Autodesk Inventor part; units mm, degrees
ref_plane "YZ Plane" through (0, 0, 0) normal (1, 0, 0) x (0, 1, 0)
ref_plane "XZ Plane" through (0, 0, 0) normal (0, 1, 0) x (-1, 0, 0)
ref_plane "XY Plane" through (0, 0, 0) normal (0, 0, 1) x (1, 0, 0)
sketch "Skizze1" plane through (0, 0, 0) normal (1, 0, 0) x (0, 1, 0)
  line L0 (12.7735, 187.5054) -> (12.7735, 177.5054) construction
  line L1 (12.7735, 177.5054) -> (95.7735, 177.5054) construction
  line L2 (95.7735, 177.5054) -> (95.7735, 203.5054) construction
  line L3 (91.4537, 203.5054) -> (93.2735, 198.5054) construction
  line L4 (95.7735, 203.5054) -> (80.7735, 203.5054) construction
  line L5 (93.2735, 198.5054) -> (83.2735, 198.5054) construction
  line L6 (83.2735, 198.5054) -> (85.0934, 203.5054) construction
  line L7 (80.7735, 203.5054) -> (80.7735, 187.5054) construction
  line L8 (80.7735, 187.5054) -> (12.7735, 187.5054) construction
  line L9 (12.7735, 187.5054) -> (12.7735, 177.5054) construction
  line L10 (15.2735, 182.5054) -> (17.0934, 187.5054) construction
  line L11 (25.2735, 182.5054) -> (15.2735, 182.5054) construction
  line L12 (23.4537, 187.5054) -> (25.2735, 182.5054) construction
  line L13 (95.7735, 177.5054) -> (95.7735, 203.4054)
  line L14 (95.7735, 203.4054) -> (91.5965, 203.4054)
  line L15 (91.5965, 203.4054) -> (93.4163, 198.4054)
  line L16 (93.4163, 198.4054) -> (83.1307, 198.4054)
  line L17 (83.1307, 198.4054) -> (84.9506, 203.4054)
  line L18 (84.9506, 203.4054) -> (80.8735, 203.4054)
  line L19 (80.8735, 203.4054) -> (80.8735, 187.4054)
  line L20 (80.8735, 187.4054) -> (23.5965, 187.4054)
  line L21 (23.5965, 187.4054) -> (25.4163, 182.4054)
  line L22 (25.4163, 182.4054) -> (15.1307, 182.4054)
  line L23 (15.1307, 182.4054) -> (16.9506, 187.4054)
  line L24 (16.9506, 187.4054) -> (12.8735, 187.4054)
  line L25 (12.8735, 187.4054) -> (12.8735, 177.5054)
  line L26 (12.8735, 177.5054) -> (95.7735, 177.5054)
  point P0 (0, 0)
  dimension "d0" = 0.1
  dimension "d1" = 0.1
  dimension "d2" = 0.1
  dimension "d3" = 0.1
  dimension "d4" = 0.1
  dimension "d5" = 0.1
  dimension "d6" = 0.1
  dimension "d7" = 0.1
extrude "Extrusion1" add sketch "Skizze1" along normal blind 7
sketch "Skizze2" plane through (0, 0, 0) normal (-1, 0, 0) x (0, 0, 1)
  line L0 (177.5054, 95.7735) -> (203.4054, 95.7735)
  line L1 (177.5054, 12.8735) -> (177.5054, 95.7735)
  line L2 (187.4054, 12.8735) -> (177.5054, 12.8735)
  line L3 (203.4054, 80.8735) -> (187.4054, 80.8735)
  line L4 (203.4054, 80.8735) -> (187.4054, 80.8735)
  line L5 (187.4054, 12.8735) -> (187.4054, 80.8735)
  line L6 (187.4054, 80.8735) -> (203.4054, 80.8735)
  line L7 (203.4054, 95.7735) -> (203.4054, 91.5965)
  line L8 (203.4054, 80.8735) -> (203.4054, 95.7735)
  point P0 (0, 0)
extrude "Extrusion2" add sketch "Skizze2" along normal blind 3.5
sketch "Skizze3" plane through (7, 0, 0) normal (1, 0, 0) x (0, 0, -1)
  line L0 (-177.5054, 95.7735) -> (-203.4054, 95.7735)
  line L1 (-177.5054, 12.8735) -> (-177.5054, 95.7735)
  line L2 (-177.5054, 12.8735) -> (-180.0054, 12.8735)
  line L3 (-187.4054, 12.8735) -> (-177.5054, 12.8735)
  line L4 (-180.0054, 12.8735) -> (-180.0054, 93.7735)
  line L5 (-177.5054, 95.7735) -> (-177.5054, 12.8735)
  line L6 (-180.0054, 93.7735) -> (-203.4054, 93.7735)
  line L7 (-203.4054, 95.7735) -> (-203.4054, 91.5965)
  line L8 (-203.4054, 93.7735) -> (-203.4054, 95.7735)
  point P0 (0, 0)
  dimension "d12" = 2.5
  dimension "d13" = 2
  dimension "d14" = 2
extrude "Extrusion3" add sketch "Skizze3" along normal blind 89.5
sketch "Skizze4" plane through (96.5, 0, 0) normal (1, 0, 0) x (0, 0, -1)
  circle A0 centre (-182.5054, 20.2735) radius 3.5 construction
  circle A1 centre (-182.5054, 88.2735) radius 3.5 construction
  circle A2 centre (-182.5054, 20.2735) radius 3.45
  circle A3 centre (-182.5054, 88.2735) radius 3.45
  point P0 (0, 0)
  dimension "d17" = 0.05
  dimension "d18" = 0.05
extrude "Extrusion4" add sketch "Skizze4" along normal blind 2
sketch "Skizze5" plane through (96.5, 0, 0) normal (1, 0, 0) x (0, 0, -1)
  line L0 (-198.9754, 90.3435) -> (-183.0054, 90.3435) construction
  line L1 (-180.0054, 17.896) -> (-180.0054, 12.8735)
  circle A0 centre (-182.5054, 88.2735) radius 3.5 construction
  line L2 (-203.4054, 93.7735) -> (-180.0054, 93.7735)
  line L3 (-180.0054, 12.8735) -> (-186.5054, 12.8735)
  line L4 (-186.5054, 12.8735) -> (-186.5054, 93.7735)
  line L5 (-186.5054, 93.7735) -> (-180.0054, 93.7735)
  line L6 (-180.0054, 93.7735) -> (-180.0054, 12.8735)
  line L7 (-203.4054, 93.7735) -> (-186.5054, 93.7735)
  line L8 (-186.5054, 93.7735) -> (-186.5054, 86.7735)
  line L9 (-186.5054, 86.7735) -> (-203.4054, 86.7735)
  line L10 (-203.4054, 86.7735) -> (-203.4054, 93.7735)
  point P0 (0, 0)
  point P1 (-186.5054, 90.3435)
  dimension "d27" = 4
  dimension "d31" = 7
extrude "Extrusion5" add sketch "Skizze5" against normal blind 7
chamfer "Fase2" distance 6.5 angle 45 1 edges at (89.5, 49.8235, 186.5054)
chamfer "Fase3" distance 6.5 angle 45 1 edges at (89.5, 86.7735, 194.9554)
equation "\"d14\" = d13"
properties part number "Batcap3"
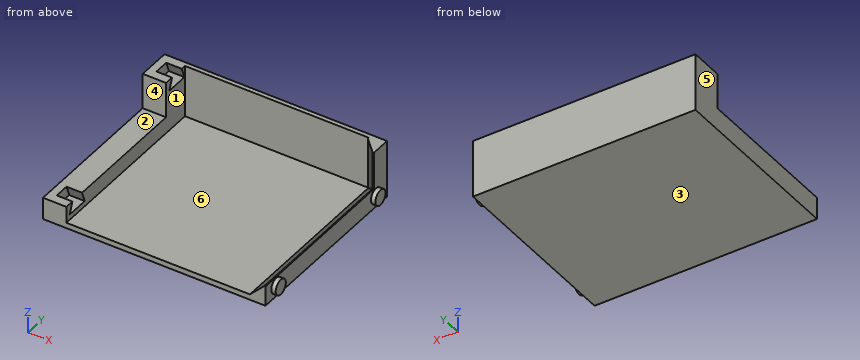
Model file for the job. Use its own axes, mm. Face numbers are marked on the shaded views. A direction names the side the tool comes from. Give positions to 0.01 mm unless a question says otherwise; leave off trailing zeros. Loops run counter-clockwise (first coordinate to the right, second up) from the corner with the lowest first, then second, coordinate; pieces in that order, holes last. Notation, with made-up numbers: (2, 54.25) -> (26, 54.25) arc R34 cw to (26, 91.25) -> close; hole circle Ø11 at (85, -30). An arc over 180 degrees is marked (long way). Use CSV: the item, a comma, the result in double quotes. Start each with the question number.
1) Slice it at A-A on z = 194.75. Give the cut face in (x, y).
2) Slice it at D-D on z = 200.75. Give the cut face in (x, y), plus the area to 3 significant figures.
3) Flat gauge pins, fed straight in: pin 1 Ø7 at (y, z) = (67.5, 187) entering from +X; pin 2 Ø3 at (x, y) = (0.5, 51) entering from +Z; pin 3 Ø0.6 at (x, z) = (96.5, 192) entering from -Y. Where does each tip first touch, or does it go through?
4) Wall check: line 1 (Y direction, x = 37, z = 188); line 2 (Z direction, x = 15, y = 90); line 3 (X direction, y = 29, z = 185.5). Give the ranges that are in metal, low to high.
5) Slice it at C-C on x = 10.5. Give the cut face in (y, z), plus the area to 3 significant figures.
6) Tool access for the marked faces 1, 2 and 3: list every direction of +Z, -Z, +X, -X, +Y, -Y with a clear straight run to the whole face (end or side of a thin tool).
7) Mould opens along X. For the marked faces 4, 5 and 6 say: released by +X, released by -X, zero draft, split by the parting line, or undercut.
Computed values:
1,outline,"(-3.5, 80.87) -> (7, 80.87) -> (7, 93.77) -> (89.5, 93.77) -> (89.5, 93.27) -> (96, 86.77) -> (96.5, 86.77) -> (96.5, 95.77) -> (-3.5, 95.77) -> close"
2,outline,"(-3.5, 80.87) -> (7, 80.87) -> (7, 83.98) -> (0, 83.98) -> (0, 92.56) -> (7, 92.56) -> (7, 93.77) -> (89.5, 93.77) -> (89.5, 93.27) -> (96, 86.77) -> (96.5, 86.77) -> (96.5, 95.77) -> (-3.5, 95.77) -> close"
2,area,"303 mm^2"
3,pin 1,"stops at x = 96.5"
3,pin 2,"stops at z = 187.41"
3,pin 3,"stops at y = 86.77"
4,line 1,"y = 93.77 to 95.77"
4,line 2,"z = 177.51 to 180.01"
4,line 3,"x = -3.5 to 7, 94.99 to 96.5"
5,outline,"(12.87, 177.51) -> (95.77, 177.51) -> (95.77, 203.41) -> (93.77, 203.41) -> (93.77, 180.01) -> (12.87, 180.01) -> close"
5,area,"254 mm^2"
6,face 1,"+Z, -Y"
6,face 2,"+Z, +X, -X, -Y"
6,face 3,"-Z, +X, -X, +Y, -Y"
7,face 4,"zero draft"
7,face 5,"released by -X"
7,face 6,"undercut"
